Geometry check sheet. Reference: the model listing, model coordinates, mm. Face numbers are marked on the shaded views. Round coordinates to 2 decimals unless told otherwise and drop trailing zeros. Order: outer loops, then holes, each group sorted by start corner. A loop starts at its lowest first (then second) coordinate and runs counter-clockwise, first axis right, second up.
(1) Draft check along X on the marked faces 1, 2 and 3. Enter one of: pulls with the +X half, pulls with the -X half, needs draft (parallel to the pull), parting line crosses it, or undercut.
(2) Gauge pin test, flat ends, axial feed: P1, Ø8, axis at x = -74.5, z = 21.5, coming from the +Y side; P2, Ø5, axis at x = -70, y = 9.5, coming from the -Z side. Record the tip position at first contact, or that the pin passes through.
(3) Cross-section at D-D on z = -35.5. Enter the section's corners in (x, y).
(4) Thickness scan on L1, parallel to X at y = 6, z = 35; L2, parallel to X at y = 25.5, z = 33. Record the ranges inside material, lowest first.
(5) Cross-section at A-A on y = 10. Enter the section's corners in (x, z).
(6) Cross-section at B-B on z = -1.5. Enter the section's corners in (x, y).
(7) Cross-section at C-C on x = -58. Enter the section's corners in (y, z).
Autodesk Inventor part; units mm, degrees
ref_plane "YZ Plane" through (0, 0, 0) normal (1, 0, 0) x (0, 1, 0)
ref_plane "XZ Plane" through (0, 0, 0) normal (0, 1, 0) x (-1, 0, 0)
ref_plane "XY Plane" through (0, 0, 0) normal (0, 0, 1) x (1, 0, 0)
sketch "스케치2" plane through (0, 0, 0) normal (0, 1, 0) x (-1, 0, 0)
  line L0 (55.5, -48.5) -> (-79.5, -48.5)
  line L1 (-79.5, -48.5) -> (-79.5, 48.5)
  line L2 (-79.5, 48.5) -> (55.5, 48.5)
  line L3 (55.5, 48.5) -> (55.5, -48.5)
  point P0 (0, 0)
  dimension "d6" = 79.5
  dimension "d7" = 48.5
  dimension "d8" = 48.5
  dimension "d9" = 55.5
extrude "돌출2" add sketch "스케치2" along normal blind 38
sketch "스케치4" plane through (0, 0, 0) normal (0, 1, 0) x (-1, 0, 0)
  line L0 (-79.5, -48.5) -> (55.5, -48.5)
  line L1 (55.5, -48.5) -> (79.5, -48.5)
  line L2 (79.5, -48.5) -> (79.5, 48.5)
  line L3 (79.5, 48.5) -> (55.5, 48.5)
  line L4 (55.5, 48.5) -> (55.5, -48.5)
  point P0 (0, 0)
  dimension "d14" = 24
extrude "돌출4" add sketch "스케치4" along normal blind 3
sketch "스케치5" plane through (0, 3, 0) normal (0, 1, 0) x (1, 0, 0)
  line L0 (-79.6369, 26.9038) -> (-63.7841, 26.9038)
  line L1 (-63.7841, 26.9038) -> (-63.7841, -41.096)
  line L2 (-63.7841, -41.096) -> (-79.6369, -41.096)
  line L3 (-79.6369, -41.096) -> (-79.6369, 26.9038)
  point P0 (0, 0)
extrude "돌출5" add sketch "스케치5" along normal blind 10
properties part number "power supply"
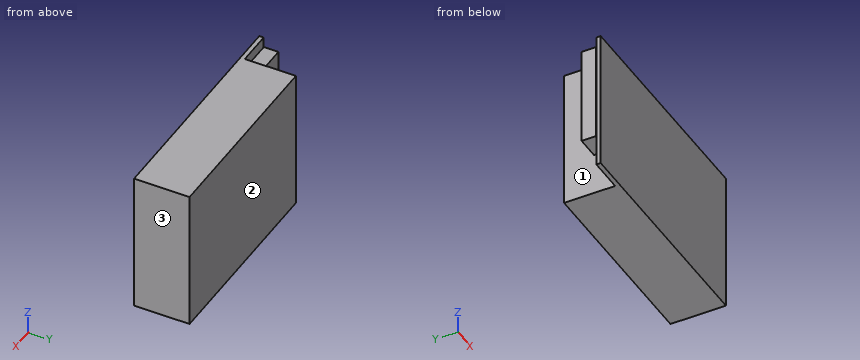
Found:
1. face 1: undercut
1. face 2: needs draft
1. face 3: pulls with the +X half
2. P1: stops at y = 13
2. P2: stops at z = -26.9
3. outline: (-79.5, 0) - (79.5, 0) - (79.5, 38) - (-55.5, 38) - (-55.5, 3) - (-79.5, 3) - close
4. L1: x = -79.64 to -63.78, -55.5 to 79.5
4. L2: x = -55.5 to 79.5
5. outline: (-79.64, -26.9) - (-63.78, -26.9) - (-63.78, 41.1) - (-79.64, 41.1) - close; (-55.5, -48.5) - (79.5, -48.5) - (79.5, 48.5) - (-55.5, 48.5) - close
6. outline: (-79.64, 3) - (-79.5, 3) - (-79.5, 0) - (79.5, 0) - (79.5, 38) - (-55.5, 38) - (-55.5, 3) - (-63.78, 3) - (-63.78, 13) - (-79.64, 13) - close
7. outline: (0, -48.5) - (3, -48.5) - (3, 48.5) - (0, 48.5) - close
